Input: part model. Units: mm. Frame: model coordinates. Face numbers are marked on the shaded views. A direction names the side the tool comes from. Give positions to 0.01 mm unless a question says otherwise; leave off trailing zeros. Loops run counter-clockwise (first coordinate to the right, second up) from the corner with the lowest first, then second, coordinate; pieces in that order, holes last. Notation, with made-up numbers: M 74.25,64.5 L 117.25,64.5 A8 cw 117.25,70.5 Z; hole C 4,33 d11. An arc over 180 degrees is marked long. Return JSON: item names as keys, results as strings. Group by question number.
```python
from build123d import *

# Parameters (mm, degrees)
SKETCH_1_W      = 582
SKETCH_1_H      = 577
EXTRUDE_1_DEPTH = 12
SKETCH_2_W      = 558
SKETCH_2_H      = 570
EXTRUDE_2_DEPTH = 580
SKETCH_3_W      = 594
SKETCH_3_H      = 589
EXTRUDE_3_DEPTH = 9


with BuildPart() as part:
    # Эскиз1 → Бобышка-Вытянуть1 (new body)
    with BuildSketch(Plane.XY):
        Rectangle(SKETCH_1_W, SKETCH_1_H)
    extrude(amount=EXTRUDE_1_DEPTH)

    # Эскиз2 → Бобышка-Вытянуть2 (add)
    with BuildSketch(Plane(origin=(0, 0, 0), x_dir=(-1, 0, 0), z_dir=(0, 0, -1))):
        with Locations((0, -9.5)):
            Rectangle(SKETCH_2_W, SKETCH_2_H)
    extrude(amount=EXTRUDE_2_DEPTH)

    # Эскиз3 → Бобышка-Вытянуть3 (add)
    with BuildSketch(Plane.XY.offset(12)):
        Rectangle(SKETCH_3_W, SKETCH_3_H)
    extrude(amount=EXTRUDE_3_DEPTH)


solid = part.part
```
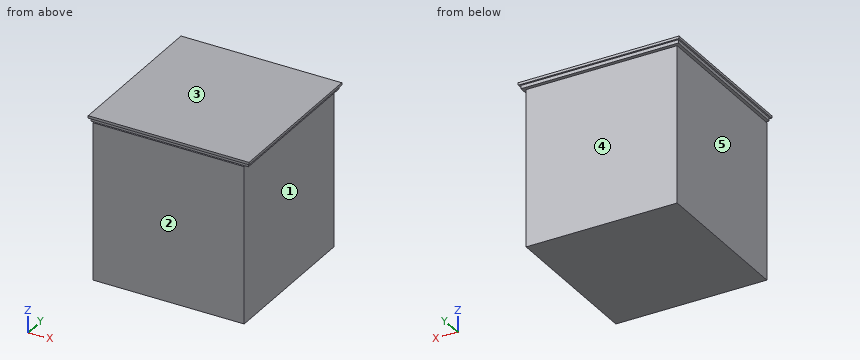
Item 1: Material intervals for line 1 (X direction, y = 271, z = -387.5); line 2 (Y direction, x = 207.5, z = -370.5), sorted ascending. Write a range as from..to.
Item 2: Section A-A, the plane x = -145.5. Return loops of the section in (y, z).
Item 3: First-contact query: pin 1 Ø1 at (y, z) = (-173.5, -432.5) entering from +X; pin 2 Ø3 at (y, z) = (71.5, -243.5) entering from -X; pin 3 Ø13 at (y, z) = (45, 5) entering from +X. Flat tips, straight axial feed; report the tip coordinate or a pass-through.
Item 4: Reachability of the marked faces 1, 2, 3, 4 and 5 from +Z, -Z, +X, -X, +Y, -Y: full face, straight path, thin tool, end or side. Return the list, or none.
Item 5: Section C-C, the plane z = -365.5. Return loops of the section in (x, y), then the cut area to 3 significant figures.
Item 6: Section B-B, the plane y = 12.5. Return loops of the section in (x, z), then the cut area to 3 significant figures.
Answer below:
{
 "1": {"line 1": "-279..279", "line 2": "-294.5..275.5"},
 "2": {"outline": "M -294.5,-580 L 275.5,-580 L 275.5,0 L 288.5,0 L 288.5,12 L 294.5,12 L 294.5,21 L -294.5,21 L -294.5,12 L -288.5,12 L -288.5,0 L -294.5,0 Z"},
 "3": {"pin 1": "x = 279", "pin 2": "x = -279", "pin 3": "x = 291"},
 "4": {"face 1": "-Z, +X, +Y, -Y", "face 2": "+Z, -Z, +X, -X, -Y", "face 3": "+Z, +X, -X, +Y, -Y", "face 4": "-Z, +X, -X, +Y", "face 5": "-Z, -X, +Y, -Y"},
 "5": {"outline": "M -279,-294.5 L 279,-294.5 L 279,275.5 L -279,275.5 Z", "area": "318,000 mm^2"},
 "6": {"outline": "M -297,12 L -291,12 L -291,0 L -279,0 L -279,-580 L 279,-580 L 279,0 L 291,0 L 291,12 L 297,12 L 297,21 L -297,21 Z", "area": "336,000 mm^2"}
}
